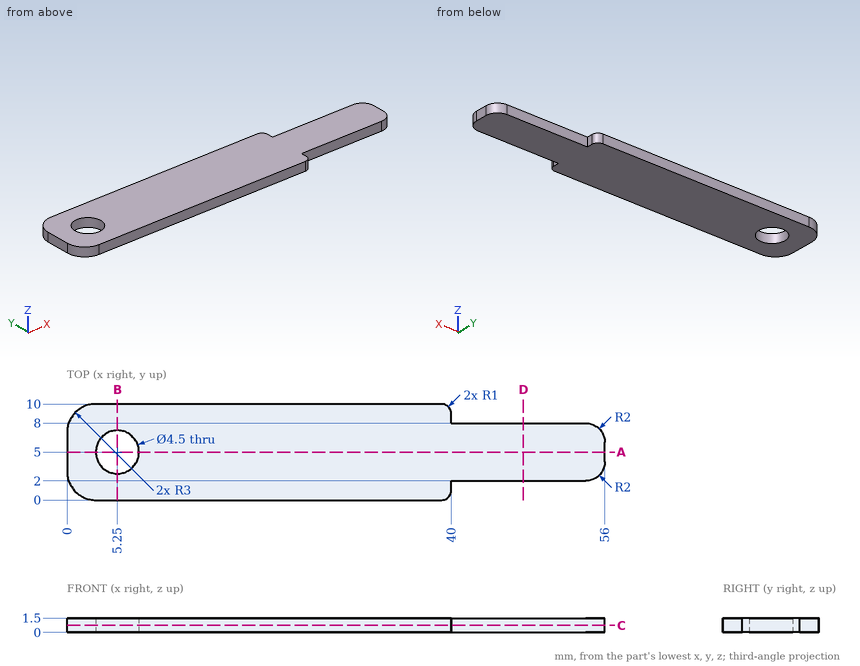
Check sheet for the drawn part. Datum: minimum x, y, z corner. Units: mm. Give positions to 0.01 mm unless a question says otherwise; leave off trailing zeros. Order: outer loops, then holes, each group sorted by start corner. A loop starts at its lowest first (then second) coordinate and runs counter-clockwise, first axis right, second up. Notation, with made-up numbers: (-7, 67.5) - (2, 67.5) arc R9 cw to (2, 72.5) - close; hole circle Ø10 at (-8, -16). An arc over 180 degrees is marked (long way). Answer as a JSON object with one key per item and string values.
(1) Depth check by flat-ended pin: pin 1 Ø2 at (x, y) = (41.5, 4.5) entering from -Z; pin 2 Ø0.8 at (x, z) = (49, 1) entering from +Y. Enter the tip coordinate at first touch or a pass-through.
Report:
{"pin 1": "z = 0", "pin 2": "y = 8"}
(2) Cross-section at D-D (x = 47.5). Record the cut outline in (y, z).
Report:
{"outline": "(2, 0) - (8, 0) - (8, 1.5) - (2, 1.5) - close"}
(3) Cross-section at C-C (z = 0.75). Record the cut outline in (x, y).
Report:
{"outline": "(0, 3) arc R3 ccw to (3, 0) - (39, 0) arc R1 ccw to (40, 1) - (40, 2) - (54, 2) arc R2 ccw to (56, 4) - (56, 6) arc R2 ccw to (54, 8) - (40, 8) - (40, 9) arc R1 ccw to (39, 10) - (3, 10) arc R3 ccw to (0, 7) - close; hole circle Ø4.5 at (5.25, 5)"}
(4) Material ranges on line 1 (Y direction, x = 5.25, z = 1.2); line 2 (X direction, y = 5.25, z = 0.25); line 3 (X direction, y = 3.25, z = 0.65), recorded low to high.
Report:
{"line 1": "0 to 2.75, 7.25 to 10", "line 2": "0 to 3.01, 7.49 to 56", "line 3": "0 to 3.84, 6.66 to 55.85"}
(5) Cross-section at B-B (x = 5.25). Record the cut outline in (y, z), then the cut area to 3 significant figures.
Report:
{"outline": "(0, 0) - (2.75, 0) - (2.75, 1.5) - (0, 1.5) - close; (7.25, 0) - (10, 0) - (10, 1.5) - (7.25, 1.5) - close", "area": "8.25 mm^2"}
(6) Cross-section at A-A (y = 5). Record the cut outline in (x, z), then the cut area to 4 significant figures.
Report:
{"outline": "(0, 0) - (3, 0) - (3, 1.5) - (0, 1.5) - close; (7.5, 0) - (56, 0) - (56, 1.5) - (7.5, 1.5) - close", "area": "77.25 mm^2"}
